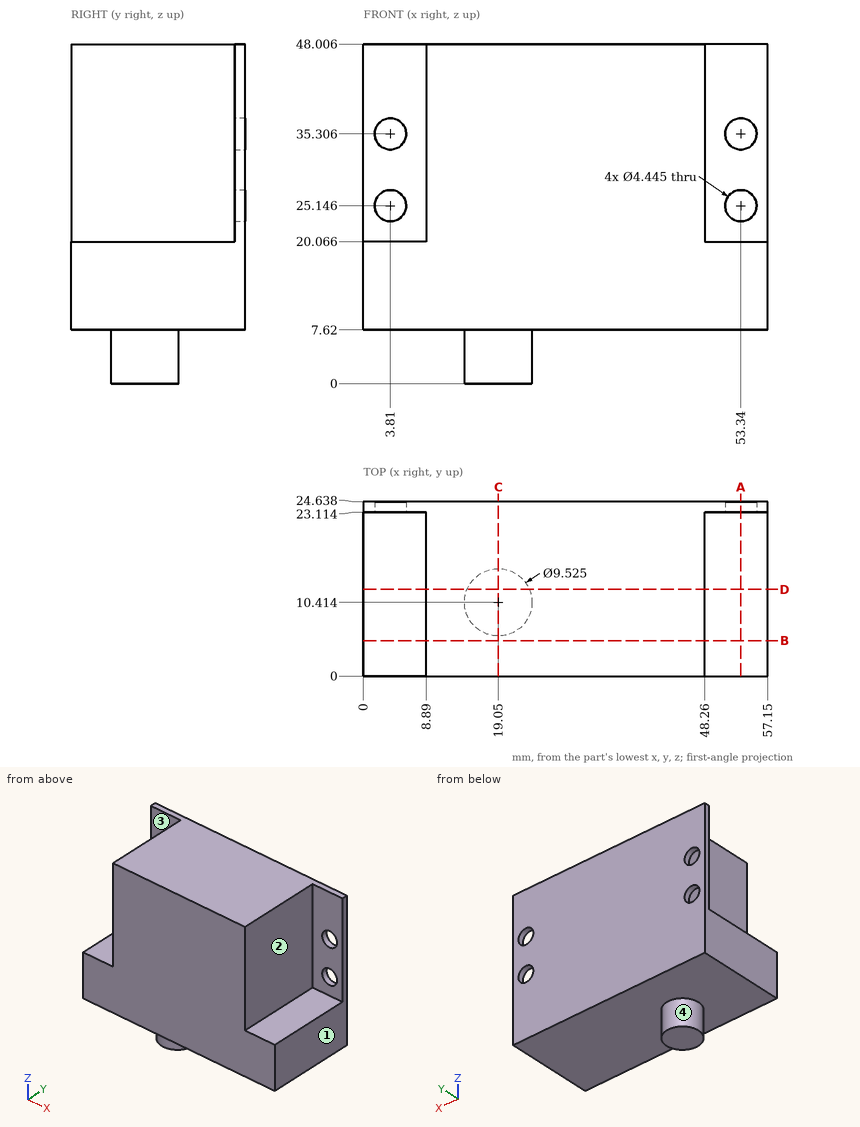
Verification items for this drawing (mm, ordinates from the low corner). A direction names the side the tool comes from. Coordinates: 2 decimals unless noted, no trailing zeros. Loops run counter-clockwise (first coordinate to the right, second up) from the corner with the lowest first, then second, coordinate; pieces in that order, holes last.
Item 1: Go/stop test with flat-tipped pins: pin 1 Ø1.5 at (y, z) = (12.5, 32) entering from -X; pin 2 Ø10 at (x, y) = (50.5, 10.5) entering from -Z; pin 3 Ø3.5 at (x, z) = (3.81, 35.306) entering from -Y; pin 4 Ø10 at (x, z) = (54.5, 31) entering from -Y. Record where each tip stops, or that it passes through.
Item 2: Sectioned sample at D-D, the plane y = 12.25. Record the boundary of the cut face in (x, z).
Item 3: Sectioned sample at A-A, the plane x = 53.34. Record the boundary of the cut face in (y, z).
Item 4: Sectioned sample at B-B, the plane y = 5. Record the boundary of the cut face in (x, z), then the cut area to 3 significant figures.
Item 5: Sectioned sample at C-C, the plane x = 19.05. Record the boundary of the cut face in (y, z), then the cut area to 3 significant figures.
Item 6: Thickness scan on line 1 (Z direction, x = 53.34, y = 23.9); line 2 (X direction, y = 5, z = 37); line 3 (Z direction, x = 30, y = 18.75). Record the ranges inside material, lowest first.
Item 7: Access from +Z, -Z, +X, -X, +Y, -Y to the whole of each face (thin tool, end or side, straight path). Record for the marked faces 1, 2, 3 and 4.
Check result:
1. pin 1: stops at x = 8.89
1. pin 2: stops at z = 7.62
1. pin 3: passes through
1. pin 4: stops at y = 23.11
2. outline: (0, 7.62) - (14.66, 7.62) - (14.66, 0) - (23.44, 0) - (23.44, 7.62) - (57.15, 7.62) - (57.15, 20.07) - (48.26, 20.07) - (48.26, 48.01) - (8.89, 48.01) - (8.89, 20.07) - (0, 20.07) - close
3. outline: (0, 7.62) - (24.64, 7.62) - (24.64, 22.92) - (23.11, 22.92) - (23.11, 20.07) - (0, 20.07) - close; (23.11, 27.37) - (24.64, 27.37) - (24.64, 33.08) - (23.11, 33.08) - close; (23.11, 37.53) - (24.64, 37.53) - (24.64, 48.01) - (23.11, 48.01) - close
4. outline: (0, 7.62) - (57.15, 7.62) - (57.15, 20.07) - (48.26, 20.07) - (48.26, 48.01) - (8.89, 48.01) - (8.89, 20.07) - (0, 20.07) - close
4. area: 1,810 mm2
5. outline: (0, 7.62) - (5.65, 7.62) - (5.65, 0) - (15.18, 0) - (15.18, 7.62) - (24.64, 7.62) - (24.64, 48.01) - (0, 48.01) - close
5. area: 1,070 mm2
6. line 1: z = 7.62 to 22.92, 27.37 to 33.08, 37.53 to 48.01
6. line 2: x = 8.89 to 48.26
6. line 3: z = 7.62 to 48.01
7. face 1: +Z, -Z, +X, +Y, -Y
7. face 2: +Z, +X, -Y
7. face 3: +Z, -X, -Y
7. face 4: -Z
